```python
from build123d import *

# Parameters (mm, degrees)
SKETCH_R        = 2.6
SKETCH_R_2      = 12.5
SKETCH_R_3      = 5.95
PAD_DEPTH       = 12
SKETCH001_W     = 42
SKETCH001_H     = 42
SKETCH001_R     = 12.5
PAD001_DEPTH    = 10
SKETCH002_R     = 1.5
POCKET_DEPTH    = 35
SKETCH003_W     = 20
SKETCH003_H     = 20
POCKET001_DEPTH = 5


with BuildPart() as part:
    # Sketch → Pad (new body)
    with BuildSketch(Plane.XY):
        with BuildLine():
            Line((32.475943, 55.828477), (32.475943, 25.828477))
            Line((32.475943, 25.828477), (35.048585, 25.828477))
            ThreePointArc((37.475943, 23.401119), (36.764986, 25.11752), (35.048585, 25.828477))
            Line((37.475943, 23.401119), (37.475943, 20.978201))
            Line((37.475943, -6.914348), (37.475943, 20.978201))
            Line((8.697616, -6.914348), (37.475943, -6.914348))
            ThreePointArc((6.370265, -5.431662), (7.317859, -6.512185), (8.697616, -6.914348))
            Line((-1.46574, 11.372705), (6.370265, -5.431662))
            ThreePointArc((-1.46574, 11.372705), (-2.398838, 12.4367), (-3.75749, 12.832711))
            Line((-21.304181, 12.832711), (-3.75749, 12.832711))
            ThreePointArc((-21.304181, 12.832711), (-22.516993, 12.479209), (-23.349932, 11.529424))
            Line((-31.707968, -6.394442), (-23.349932, 11.529424))
            ThreePointArc((-32.524057, -6.914348), (-32.040243, -6.773329), (-31.707968, -6.394442))
            Line((-62.524057, -6.914348), (-32.524057, -6.914348))
            Line((-62.524057, 17.407665), (-62.524057, -6.914348))
            Line((-62.524057, 17.407665), (-62.524057, 24.589269))
            ThreePointArc((-60.707672, 26.405654), (-61.99205, 25.873647), (-62.524057, 24.589269))
            Line((-60.707672, 26.405654), (-57.524057, 26.405654))
            Line((-57.524057, 26.405654), (-57.524057, 56.405654))
            Line((-57.524057, 56.405654), (-38.879514, 56.405654))
            ThreePointArc((-38.879514, 56.405654), (-37.835318, 56.838174), (-37.402798, 57.882371))
            Line((-37.402798, 57.882371), (-37.402798, 63.120448))
            ThreePointArc((-34.836585, 65.686661), (-36.651171, 64.935034), (-37.402798, 63.120448))
            Line((-34.836585, 65.686661), (9.286369, 65.686661))
            ThreePointArc((11.852582, 63.120448), (11.100956, 64.935034), (9.286369, 65.686661))
            Line((11.852582, 63.120448), (11.852582, 57.305194))
            ThreePointArc((11.852582, 57.305194), (12.285103, 56.260997), (13.329299, 55.828477))
            Line((13.329299, 55.828477), (32.475943, 55.828477))
        make_face()
        with Locations((-50.024057, 6.023385)):
            Circle(SKETCH_R, mode=Mode.SUBTRACT)
        with Locations((-32.024057, 6.023385)):
            Circle(SKETCH_R, mode=Mode.SUBTRACT)
        with Locations((24.975943, 5.585652)):
            Circle(SKETCH_R, mode=Mode.SUBTRACT)
        with Locations((6.975943, 5.585652)):
            Circle(SKETCH_R, mode=Mode.SUBTRACT)
        with Locations((-12.524057, 41.405654)):
            Circle(SKETCH_R_2, mode=Mode.SUBTRACT)
        with Locations((-37.024057, 41.405654)):
            Circle(SKETCH_R_3, mode=Mode.SUBTRACT)
        with Locations((11.975943, 40.828477)):
            Circle(SKETCH_R_3, mode=Mode.SUBTRACT)
    extrude(amount=PAD_DEPTH)

    # Sketch001 (on Face36 of Pad) → Pad001 (join)
    with BuildSketch(Plane(origin=(0, 0, 0), x_dir=(1, 0, 0), z_dir=(0, 0, -1))):
        with Locations((-12.524057, -41.405654)):
            Rectangle(SKETCH001_W, SKETCH001_H)
        with Locations((-12.524057, -41.405654)):
            Circle(SKETCH001_R, mode=Mode.SUBTRACT)
    extrude(amount=PAD001_DEPTH)

    # Sketch002 (on Face43 of Pad001) → Pocket (cut)
    with BuildSketch(Plane(origin=(0, 0, -10), x_dir=(1, 0, 0), z_dir=(0, 0, -1))):
        with Locations((-27.524057, -26.405654)):
            Circle(SKETCH002_R)
        with Locations((2.475943, -26.405654)):
            Circle(SKETCH002_R)
        with Locations((2.475943, -56.405654)):
            Circle(SKETCH002_R)
        with Locations((-27.524057, -56.405654)):
            Circle(SKETCH002_R)
    extrude(amount=-POCKET_DEPTH, mode=Mode.SUBTRACT)

    # Sketch003 (on Face5 of Pocket) → Pocket001 (cut)
    with BuildSketch(Plane.XY.offset(12)):
        with Locations((-50.024057, 6.023385)):
            Rectangle(SKETCH003_W, SKETCH003_H)
        with Locations((24.975943, 5.585652)):
            Rectangle(SKETCH003_W, SKETCH003_H)
    extrude(amount=-POCKET001_DEPTH, mode=Mode.SUBTRACT)


solid = part.part
```
For this review, take the finished solid that the model builds, in its own axes (mm). A direction names the side the tool comes from. Give positions to 0.01 mm unless a question says otherwise; leave off trailing zeros. Write each loop counter-clockwise with the first axis right and the second up, starting at its lowest first coordinate (ties: lowest second). Pieces come first, ordered by that corner, then holes. Notation, with made-up numbers: M 15.25,55 L 57.25,55 A25 cw 57.25,73 Z; hole C 4.5,23 d11. An arc over 180 degrees is marked long. Answer as a JSON object with one key per item and string values. Group by question number.
Item 1: For pin 1 Ø4 at (y, z) = (61.5, 9) entering from -X; pin 2 Ø6 at (x, y) = (6.98, 5.59) entering from -Z; pin 3 Ø2.5 at (x, y) = (-27.52, 56.41) entering from -Z; pin 4 Ø1.5 at (x, z) = (-51, 9.5) entering from +Y, all flat-tipped, find the tip position at first contact; note any pin that passes through.
Item 2: Consider section D-D on z = -3. Write out the cut boundary in (x, y), plus the area to 3 significant figures.
Item 3: Tool access review of faces 1 (the flat face through (-13, 12.833, 6)), 2 (the flat face through (8.476, 42, -5)), 3 (the flat face through (25, 15.586, 10)), 4 (the flat face through (-13, 20.406, -5)): name each direction out of +Z, -Z, +X, -X, +Y, -Y from which nothing blocks a thin tool from reaching the whole face with its end or side.
Item 4: For probe 1 along Y at (x, z) = (-28, -8.5); probe 2 along X at (y, z) = (55.5, -7); probe 3 along Z at (x, y) = (-55.5, 26), list the stretches that pass through material, from the lowest coordinate up. Write a range as [from, to].
Item 5: Consider section A-A on x = 20. Write out the cut boundary in (y, z), plus the area to 3 significant figures.
Item 6: Consider section C-C on x = -6. Write out the cut boundary in (y, z), plus the area to 3 significant figures.
Item 7: Draft analysis for pull direction Y (two halves, no side actions). For faces 5 (the cylindrical face through (7.3, -6.5, 5.9)), 6 (the flat face through (32.476, 41, 6)), 7 (the flat face through (-50, 16.023, 10)), state which applies: +Y half, -Y half, draft (parallel to the pull), parting line (faces both ways), or undercut.
Item 8: Consider section B-B on y = 33. Write out the cut boundary in (x, z), plus the area to 3 significant figures.
Check result:
{
 "1": {"pin 1": "stops at x = -37.4", "pin 2": "stops at z = 0", "pin 3": "passes through", "pin 4": "stops at y = 56.41"},
 "2": {"outline": "M -33.52,20.41 L 8.48,20.41 L 8.48,62.41 L -33.52,62.41 Z; hole C -27.52,26.41 d3; hole C -27.52,56.41 d3; hole C -12.52,41.41 d25; hole C 2.48,26.41 d3; hole C 2.48,56.41 d3", "area": "1,240 mm^2"},
 "3": {"face 1": "+Z, -Z, -Y", "face 2": "-Z, +X, +Y, -Y", "face 3": "+Z", "face 4": "-Z, +X, -X, -Y"},
 "4": {"probe 1": "y = [20.41, 24.98], [27.83, 54.98], [57.83, 62.41]", "probe 2": "x = [-33.52, -28.72], [-26.33, 1.28], [3.67, 8.48]", "probe 3": "z = [0, 12]"},
 "5": {"outline": "M -6.91,0 L 55.83,0 L 55.83,12 L 15.59,12 L 15.59,7 L -4.41,7 L -4.41,12 L -6.91,12 Z", "area": "653 mm^2"},
 "6": {"outline": "M 12.83,0 L 20.41,0 L 20.41,-10 L 30.74,-10 L 30.74,12 L 12.83,12 Z; M 52.07,-10 L 62.41,-10 L 62.41,0 L 65.69,0 L 65.69,12 L 52.07,12 Z", "area": "585 mm^2"},
 "7": {"face 5": "-Y half", "face 6": "draft", "face 7": "undercut"},
 "8": {"outline": "M -57.52,0 L -33.52,0 L -33.52,-10 L -21.78,-10 L -21.78,12 L -57.52,12 Z; M -3.27,-10 L 8.48,-10 L 8.48,0 L 32.48,0 L 32.48,12 L -3.27,12 Z", "area": "1,090 mm^2"}
}
